For this review, use the dimensioned drawing (mm, ordinates from the lowest corner) and the shaded views. A direction names the side the tool comes from. Give positions to 0.01 mm unless a question says otherwise; leave off trailing zeros. Loops run counter-clockwise (first coordinate to the right, second up) from the corner with the lowest first, then second, coordinate; pieces in that order, holes last. Notation, with made-up numbers: M 80,10.25 L 90,10.25 A17 ccw 90,15.25 Z; hole C 29,87.25 d10. An arc over 180 degrees is marked long. Return JSON: item names as keys, results as strings.
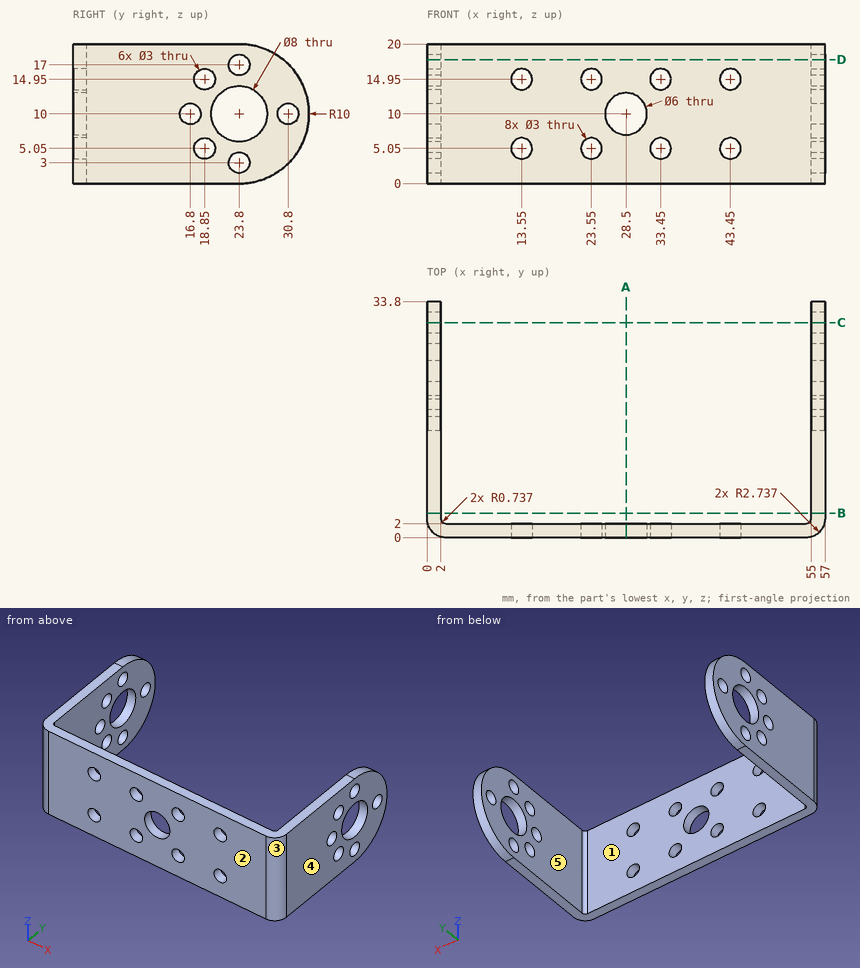
1) Tool access review of the marked faces 4 and 5: name each direction out of +Z, -Z, +X, -X, +Y, -Y from which nothing blocks a thin tool from reaching the whole face with its end or side.
From the geometry:
{"face 4": "+Z, -Z, +X, +Y, -Y", "face 5": "+Z, -Z, +Y"}
2) Consider section B-B on y = 3.5. Write out the cut boundary in (x, z).
From the geometry:
{"outline": "M 0,0 L 2,0 L 2,20 L 0,20 Z; M 55,0 L 57,0 L 57,20 L 55,20 Z"}
3) Wall thickness on L1, parallel to X at y = 22.5, z = 4; L2, parallel to Y at x = 56.4, z = 10 (1 decimal); L3, parallel to Y at x = 21.5, z = 13.5: over which ranges is each line inside the solid? List them lowest first. Write a range as from..to.
From the geometry:
{"L1": "0..2, 55..57", "L2": "1..15.3, 18.3..19.8, 27.8..29.3, 32.3..33.8", "L3": "0..2"}
4) Consider section C-C on y = 30.8. Write out the cut boundary in (x, z).
From the geometry:
{"outline": "M 0,2.86 L 2,2.86 L 2,8.5 L 0,8.5 Z; M 0,11.5 L 2,11.5 L 2,17.14 L 0,17.14 Z; M 55,2.86 L 57,2.86 L 57,8.5 L 55,8.5 Z; M 55,11.5 L 57,11.5 L 57,17.14 L 55,17.14 Z"}
5) Insertion check: pin 1 (4 mm diameter, centred on x = 33.45, z = 5.05, fed in from +Y). The pin has a flat end and moves straight along its axis. Give the tip position at first contact, or say it passes through.
From the geometry:
{"pin 1": "y = 2"}
6) Consider section A-A on x = 28.5. Write out the cut boundary in (y, z), then the cut area to 3 significant figures.
From the geometry:
{"outline": "M 0,0 L 2,0 L 2,7 L 0,7 Z; M 0,13 L 2,13 L 2,20 L 0,20 Z", "area": "28.0 mm²"}
7) The part is to be moulded in two halves that separate along X. For the marked faces 1, 2 and 3, say which applies: released by +X, released by -X, zero draft, split by the parting line, or undercut.
From the geometry:
{"face 1": "undercut", "face 2": "zero draft", "face 3": "released by +X"}
8) Consider section D-D on z = 17.75. Write out the cut boundary in (x, y).
From the geometry:
{"outline": "M 0,2.74 A2.74 ccw 2.74,0 L 54.26,0 A2.74 ccw 57,2.74 L 57,22.5 L 55,22.5 L 55,2.74 A0.74 cw 54.26,2 L 2.74,2 A0.74 cw 2,2.74 L 2,22.5 L 0,22.5 Z; M 0,25.1 L 2,25.1 L 2,30.12 L 0,30.12 Z; M 55,25.1 L 57,25.1 L 57,30.12 L 55,30.12 Z"}
